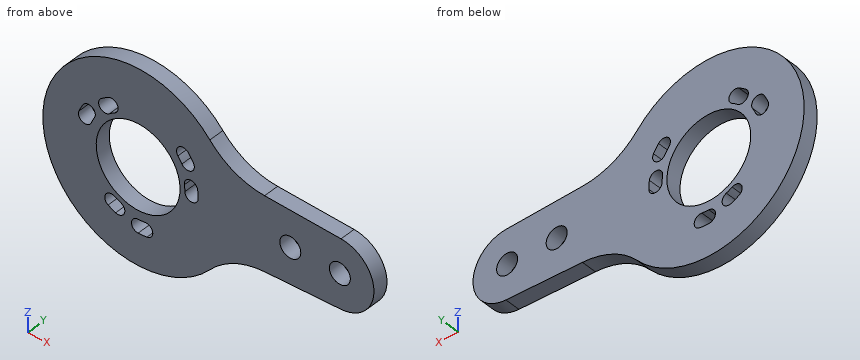
from build123d import *

# Parameters (mm, degrees)
BOSS_EXTRUDE1_DEPTH = 4
FILLET1_R           = 20
SKETCH1_R           = 11
SKETCH1_R_2         = 2.75
CUT_EXTRUDE3_DEPTH  = 131.855321132


with BuildPart() as part:
    # Sketch3 → Boss-Extrude1 (new body)
    with BuildSketch(Plane(origin=(0, 0, 0), x_dir=(1, 0, 0), z_dir=(0, 1, 0))):
        with BuildLine():
            Line((22.912878475, 10), (53.225121597, 8.941473145))
            ThreePointArc((53.225121597, 8.941473145), (61.859801844, 0), (53.225121597, -8.941473145))
            Line((53.225121597, -8.941473145), (22.912878475, -10))
            ThreePointArc((22.912878475, -10), (-25, 0), (22.912878475, 10))
        make_face()
    extrude(amount=BOSS_EXTRUDE1_DEPTH)

    # Fillet1
    fillet1_edges = [part.edges().sort_by_distance(p)[0] for p in [
        (22.912878475, 2, -10),
        (22.912878475, 2, 10),
    ]]
    fillet(fillet1_edges, radius=FILLET1_R)

    # Sketch1 → Cut-Extrude3 (cut, through all)
    with BuildSketch(Plane(origin=(103.38268991, 0, 0), x_dir=(1, 0, 0), z_dir=(0, 1, 0))):
        with Locations(Location((-103.38268991, 0, 0), (0, 0, 270))):
            Circle(SKETCH1_R)
        with Locations(Location((-63.469811435, 0, 0), (0, 0, 90))):
            Circle(SKETCH1_R_2)
        with Locations(Location((-50.469811435, 0, 0), (0, 0, 90))):
            Circle(SKETCH1_R_2)
        with BuildLine():
            ThreePointArc((-111.25768991, 13.63990011), (-110.287035472, 14.156006229), (-109.282743756, 14.603145709))
            ThreePointArc((-109.282743756, 14.603145709), (-107.004610472, 13.636135502), (-107.971620679, 11.358002218))
            ThreePointArc((-107.971620679, 11.358002218), (-108.752736458, 11.010227067), (-109.50768991, 10.608811196))
            ThreePointArc((-109.50768991, 10.608811196), (-111.898234366, 11.249355653), (-111.25768991, 13.63990011))
        make_face()
        with BuildLine():
            ThreePointArc((-101.538646322, 13.121051911), (-102.458416633, 13.217723666), (-103.38268991, 13.25))
            ThreePointArc((-103.38268991, 13.25), (-105.13268991, 15), (-103.38268991, 16.75))
            ThreePointArc((-103.38268991, 16.75), (-102.214268974, 16.709197842), (-101.051540469, 16.586990151))
            ThreePointArc((-101.051540469, 16.586990151), (-99.562124275, 14.610468104), (-101.538646322, 13.121051911))
        make_face()
        with BuildLine():
            ThreePointArc((-87.63268991, 0), (-89.38268991, 1.75), (-91.13268991, 0))
            ThreePointArc((-91.13268991, 0), (-91.162530294, -0.854516803), (-91.251906068, -1.704870487))
            ThreePointArc((-91.251906068, -1.704870487), (-89.762489874, -3.681392534), (-87.785967827, -2.19197634))
            ThreePointArc((-87.785967827, -2.19197634), (-87.671056118, -1.098664461), (-87.63268991, 0))
        make_face()
        with BuildLine():
            ThreePointArc((-92.941547424, -8.157514548), (-92.639936187, -10.613940949), (-90.183509787, -10.312329712))
            ThreePointArc((-90.183509787, -10.312329712), (-89.496310569, -9.366481133), (-88.876764396, -8.375))
            ThreePointArc((-88.876764396, -8.375), (-89.517308853, -5.984455543), (-91.90785331, -6.625))
            ThreePointArc((-91.90785331, -6.625), (-92.397942073, -7.409305971), (-92.941547424, -8.157514548))
        make_face()
        with BuildLine():
            ThreePointArc((-111.25768991, -13.63990011), (-108.867145453, -12.999355653), (-109.50768991, -10.608811196))
            ThreePointArc((-109.50768991, -10.608811196), (-110.232802977, -10.155710264), (-110.924542982, -9.653131732))
            ThreePointArc((-110.924542982, -9.653131732), (-113.380969383, -9.954742969), (-113.079358146, -12.411169369))
            ThreePointArc((-113.079358146, -12.411169369), (-112.189978139, -13.057341768), (-111.25768991, -13.63990011))
        make_face()
        with BuildLine():
            ThreePointArc((-115.667875983, -4.963537363), (-117.946009267, -3.996527156), (-118.913019474, -6.27466044))
            ThreePointArc((-118.913019474, -6.27466044), (-118.437490185, -7.342716709), (-117.888615423, -8.375))
            ThreePointArc((-117.888615423, -8.375), (-115.498070966, -9.015544457), (-114.85752651, -6.625))
            ThreePointArc((-114.85752651, -6.625), (-115.291711023, -5.808417695), (-115.667875983, -4.963537363))
        make_face()
    extrude(amount=CUT_EXTRUDE3_DEPTH, mode=Mode.SUBTRACT)


solid = part.part
The listing builds one solid part. Answer for the finished solid, in the listing's coordinates (mm). Round coordinates to 2 decimals unless told otherwise and drop trailing zeros. Order: outer loops, then holes, each group sorted by start corner. A loop starts at its lowest first (then second) coordinate and runs counter-clockwise, first axis right, second up. Notation, with made-up numbers: (66.25, 83) -> (89.25, 83) arc R23 cw to (89.25, 119) -> close; hole circle Ø11 at (10, 74.25). An arc over 180 degrees is marked (long way). Put each result on its own line as item: value.
Q1. Consider line 1 along Z through (x, y) = (0, 2.05); line 2 along X through (y, z) = (3.35, 0.5) (3 decimals); line 3 along Z through (x, y) = (-0.5, 1.35) (3 decimals). Determine where each line is inside the solid, lowest interval first.
Results list:
line 1: -25 to -16.75, -13.25 to -11, 11 to 25
line 2: -24.995 to -10.989, 10.989 to 12.24, 15.742 to 37.209, 42.617 to 50.209, 55.617 to 61.846
line 3: -24.995 to -16.677, -13.323 to -10.989, 10.989 to 24.995
Q2. Section C-C, the plane z = -18.5 is taken. Write down the section's boundary in (x, y), and give its area (3 significant figures).
Results list:
outline: (-16.82, 0) -> (16.82, 0) -> (16.82, 4) -> (-16.82, 4) -> close
area: 135 mm^2
Q3. Section A-A, the plane y = 1.75 is taken. Count the separate pieces of the cut face and the enclosed holes in it, and give its area (3 significant figures).
Results list:
separate pieces: 1
enclosed holes: 9
area: 2,130 mm^2
Q4. Section B-B, the plane z = -6.5 is taken. Write down the section's boundary in (x, y).
Results list:
outline: (-24.14, 0) -> (-8.87, 0) -> (-8.87, 4) -> (-24.14, 4) -> close; (8.87, 0) -> (59.06, 0) -> (59.06, 4) -> (8.87, 4) -> close
Q5. Each of these flat-tipped pins is pushed along its axis until it touches: P1, Ø6, axis at x = 0, z = 18, coming from the -Y side; P2, Ø2, axis at x = 22, y = 2, coming from the -Z side; P3, Ø1.5, axis at x = 20.5, y = 3, coming from the +Z side; P4, Ø17.5, axis at x = 0, z = 0, coming from the +Y side. Where does it stop, or does it pass through?
Results list:
P1: y = 0
P2: z = -14.32
P3: z = 15.46
P4: through
